Input: part model. Units: mm. Frame: model coordinates. A direction names the side the tool comes from. Coordinates: 2 decimals unless noted, no trailing zeros. Loops run counter-clockwise (first coordinate to the right, second up) from the corner with the lowest first, then second, coordinate; pieces in that order, holes last.
```python
from build123d import *

# Parameters (mm, degrees)
BOX003_W               = 3.325
BOX003_H               = 3.325
BOX003_DEPTH           = 19.325
CYLINDER002_R          = 1.5
CYLINDER002_DEPTH      = 19.325
BOX005_W               = 0.455
BOX005_H               = 2.325
BOX005_DEPTH           = 16.625
BOX004_W               = 0.455
BOX004_H               = 2.325
BOX004_DEPTH           = 16.625
CYLINDER001_R          = 2.6625
CYLINDER001_DEPTH      = 26.75
CYLINDER_R             = 6.1625
CYLINDER_DEPTH         = 15.825
BOX_W                  = 12.325
BOX_H                  = 10.325
BOX_DEPTH              = 15.825
BOX002_W               = 12.325
BOX002_H               = 10.325
BOX002_DEPTH           = 9.325
FUSION_PLACEMENT_ANGLE = 180


with BuildPart() as cube003:
    # Box003 → Box003 (new body)
    with BuildSketch(Plane(origin=(-1.6625, 0.8375, 0), x_dir=(1, 0, 0), z_dir=(0, 0, 1))):
        with Locations((1.6625, 1.6625)):
            Rectangle(BOX003_W, BOX003_H)
    extrude(amount=BOX003_DEPTH)


with BuildPart() as shaft:
    # Cylinder002 → Cylinder002 (new body)
    with BuildSketch(Plane.XY):
        Circle(CYLINDER002_R)
    extrude(amount=CYLINDER002_DEPTH)

    # Cut: cut Cube003
    add(cube003.part, mode=Mode.SUBTRACT)


with BuildPart() as cube005:
    # Box005 → Box005 (new body)
    with BuildSketch(Plane(origin=(-3.4775, -1.1625, -16.625), x_dir=(1, 0, 0), z_dir=(0, 0, 1))):
        with Locations((0.2275, 1.1625)):
            Rectangle(BOX005_W, BOX005_H)
    extrude(amount=BOX005_DEPTH)


with BuildPart() as contacts:
    # Box004 → Box004 (new body)
    with BuildSketch(Plane(origin=(3.0225, -1.1625, -16.625), x_dir=(1, 0, 0), z_dir=(0, 0, 1))):
        with Locations((0.2275, 1.1625)):
            Rectangle(BOX004_W, BOX004_H)
    extrude(amount=BOX004_DEPTH)

    # Fusion001: union Cube005
    add(cube005.part)


with BuildPart() as cylinder001:
    # Cylinder001 → Cylinder001 (new body)
    with BuildSketch(Plane.XY.offset(-10.125)):
        Circle(CYLINDER001_R)
    extrude(amount=CYLINDER001_DEPTH)


with BuildPart() as cylinder:
    # Cylinder → Cylinder (new body)
    with BuildSketch(Plane.XY):
        Circle(CYLINDER_R)
    extrude(amount=CYLINDER_DEPTH)


with BuildPart() as common:
    # Box → Box (new body)
    with BuildSketch(Plane(origin=(-6.1625, -5.1625, 0), x_dir=(1, 0, 0), z_dir=(0, 0, 1))):
        with Locations((6.1625, 5.1625)):
            Rectangle(BOX_W, BOX_H)
    extrude(amount=BOX_DEPTH)

    # Common: intersect Cylinder
    add(cylinder.part, mode=Mode.INTERSECT)


with BuildPart() as n20gearedmotor:
    # Box002 → Box002 (new body)
    with BuildSketch(Plane(origin=(-6.1625, -5.1625, -9.325), x_dir=(1, 0, 0), z_dir=(0, 0, 1))):
        with Locations((6.1625, 5.1625)):
            Rectangle(BOX002_W, BOX002_H)
    extrude(amount=BOX002_DEPTH)

    # Fusion: union Cylinder001, Common
    add(cylinder001.part)
    add(common.part)


with BuildPart() as n20gearedmotor_1:
    # Fusion placement: moved
    add(n20gearedmotor.part.rotate(Axis((0, 0, 0), (1, 0, 0)), FUSION_PLACEMENT_ANGLE))

    # Fusion002: union Shaft, Contacts
    add(shaft.part)
    add(contacts.part)


solid = n20gearedmotor_1.part
```
Item 1: Mould query, pull axis X, two halves, no side actions, for faces 5 (the face through (-3.022, 0, -16)), 6 (the face through (6.162, 0, 5)), 7 (the face through (-5, -4, 0)). Classes: +X half, -X half, draft (parallel to the pull), parting line (faces both ways), or undercut.
Result:
face 5: undercut
face 6: +X half
face 7: draft
Item 2: Contact query for flat-ended pins moving along their axis: P1, Ø3, axis at x = -5.5, y = 2, coming from the -Z side (3 decimals); P2, Ø2.5, axis at x = 0.5, z = 16.5, coming from the +Y side; P3, Ø1.5, axis at y = 1.5, z = -7.5, coming from the +X side. Output: stop coordinate, or through.
Result:
P1: stops at z = -15.825
P2: stops at y = 0.84
P3: stops at x = 6.12
Item 3: Line query: L1, parallel to Z at x = 4.75, y = 4.5 (3 decimals); L2, parallel to Z at x = 5, y = -0.5 (3 decimals); L3, parallel to X at y = 4.25, z = -6. Output: solid intervals per line, ascending.
Result:
L1: z = 0 to 9.325
L2: z = -15.825 to 9.325
L3: x = -4.46 to 4.46
Item 4: Section query A-A (x = 0). Output: boundary loops of the cut face in (y, z) (1 decimal).
Result:
outline: (-5.2, -15.8) - (-2.7, -15.8) - (-2.7, -16.6) - (2.7, -16.6) - (2.7, -15.8) - (5.2, -15.8) - (5.2, 9.3) - (2.7, 9.3) - (2.7, 10.1) - (0.8, 10.1) - (0.8, 19.3) - (-1.5, 19.3) - (-1.5, 10.1) - (-2.7, 10.1) - (-2.7, 9.3) - (-5.2, 9.3) - close
Item 5: Section query C-C (z = -4.5). Output: boundary loops of the cut face in (x, y) (1 decimal).
Result:
outline: (-3.4, -5.2) - (3.4, -5.2) arc R6.2 ccw to (3.4, 5.2) - (-3.4, 5.2) arc R6.2 ccw to start
Item 6: Section query D-D (x = -4.75). Output: boundary loops of the cut face in (y, z) (1 decimal).
Result:
outline: (-5.2, 0) - (-3.9, 0) - (-3.9, -15.8) - (3.9, -15.8) - (3.9, 0) - (5.2, 0) - (5.2, 9.3) - (-5.2, 9.3) - close
Item 7: Section query B-B (y = 4). Output: boundary loops of the cut face in (x, z) (1 decimal).
Result:
outline: (-6.2, 0) - (-4.7, 0) - (-4.7, -15.8) - (4.7, -15.8) - (4.7, 0) - (6.2, 0) - (6.2, 9.3) - (-6.2, 9.3) - close
Item 8: Reachability of faces 1 (the face through (0, 0.837, 15)), 2 (the face through (5, -4, 0)), 3 (the face through (-1.5, -2.4, 9.325)), 4 (the face through (-5, 4, 0)) from +Z, -Z, +X, -X, +Y, -Y: full face, straight path, thin tool, end or side. Return the list, or none.
Result:
face 1: +Z, +X, -X, +Y
face 2: -Z, +X, -Y
face 3: +Z
face 4: -Z, -X, +Y
